Autodesk Inventor part; units mm, degrees
ref_plane "YZ Plane" through (0, 0, 0) normal (1, 0, 0) x (0, 1, 0)
ref_plane "XZ Plane" through (0, 0, 0) normal (0, 1, 0) x (-1, 0, 0)
ref_plane "XY Plane" through (0, 0, 0) normal (0, 0, 1) x (1, 0, 0)
sketch "Sketch1" plane through (0, 0, 0) normal (0, 0, 1) x (1, 0, 0)
  arc A0 (-5, -2.9) -> (-4.8506, -3.2565) centre (-4.5, -2.9) ccw
  line L0 (-5, -2.6) -> (-5, -2.9)
  arc A1 (-4.5, -2.1) -> (-5, -2.6) centre (-4.5, -2.6) ccw
  line L1 (-4.8506, -3.2565) -> (-1.8506, -6.2065)
  arc A2 (-1.8506, -6.2065) -> (-1.5, -6.35) centre (-1.5, -5.85) ccw
  line L2 (-1.5, -6.35) -> (1.5, -6.35)
  line L3 (4.5, -2.1) -> (-4.5, -2.1)
  arc A3 (1.5, -6.35) -> (1.8506, -6.2065) centre (1.5, -5.85) ccw
  line L4 (4.8506, -3.2565) -> (1.8506, -6.2065)
  arc A4 (5, -2.6) -> (4.5, -2.1) centre (4.5, -2.6) ccw
  arc A5 (4.8506, -3.2565) -> (5, -2.9) centre (4.5, -2.9) ccw
  line L5 (5, -2.6) -> (5, -2.9)
  line L6 (-2.5, 0) -> (2.5, 0)
  line L7 (-2.5, 0) -> (-2.5, -2.1)
  line L8 (2.5, 0) -> (2.5, -2.1)
  point P0 (0, -6.35)
  point P1 (0, 0)
  point P2 (0, -2.1)
  point P3 (0, 0)
  dimension "d9" = 4.25
  dimension "d10" = 10
  dimension "d12" = 0.3
  dimension "d13" = 9
  dimension "d14" = 3
  dimension "d17" = 2.1
  dimension "d18" = 5
extrude "Extrusion1" add sketch "Sketch1" along normal blind 8
sketch "Sketch2" plane through (0, 0, 0) normal (0, 0, -1) x (-1, 0, 0)
  line L0 (-2.5, 0) -> (2.5, 0)
  line L1 (2.5, 0) -> (12, 0)
  line L2 (-2.5, -2.1) -> (-2.5, 0)
  line L3 (12, 0) -> (3.3532, 8.6468)
  line L4 (-0.6066, 4.687) -> (2.0804, 2)
  line L5 (3.3532, 8.6468) -> (-0.6066, 4.687)
  line L6 (2.0804, 2) -> (6.0402, 5.9598)
  line L7 (10, 0) -> (10, 2)
  line L8 (3.3532, 8.6468) -> (1.2319, 10.7681)
  line L9 (1.2319, 10.7681) -> (-4.8492, 4.687)
  line L10 (-4.8492, 4.687) -> (-2.5, 0)
  point P0 (0, 0)
  dimension "d21" = 12
  dimension "d23" = 45
  dimension "d24" = 3.8
  dimension "d25" = 5.6
  dimension "d26" = 2
  dimension "d28" = 3
  dimension "d34" = 10
extrude "Extrusion2" add sketch "Sketch2" against normal up to surface (8 mm away) contours L10 L9 L8 L5 L4 L6 L3 L7 L1 L0 | L3 L6 L4 L5
sketch "Sketch3" plane through (-1.2319, 10.7681, 0) normal (-0.7071, 0.7071, 0) x (-0.7071, -0.7071, 0)
  line L0 (12.4, 0) -> (12.4, 8)
  line L1 (6.8, 0) -> (3, 0)
  line L2 (12.4, 0) -> (0, 0)
  circle A0 centre (4.9, 4) radius 1.9
  point P0 (6.7431, 0)
  point P1 (12.4, 4)
  point P2 (4.9, 0)
  dimension "d31" = 3.8
extrude "Extrusion3" cut sketch "Sketch3" against normal blind 5.6
properties part number "Profil-ElBoardHold"
The listing builds one solid part. Answer for the finished solid, in the listing's coordinates (mm). A direction names the side the tool comes from. Give positions to 0.01 mm unless a question says otherwise; leave off trailing zeros. Write each loop counter-clockwise with the first axis right and the second up, starting at its lowest first coordinate (ties: lowest second). Pieces come first, ordered by that corner, then holes. Notation, with made-up numbers: (-16.75, 4) - (6.25, 4) arc R17 cw to (6.25, 33) - close; hole circle Ø1 at (39, 30.25). An arc over 180 degrees is marked (long way). Use a Markdown table: item, result.
1. Section A-A on z = 7.5 is taken. Write down the section's boundary in (x, y).
Values follow:
| item | result |
|---|---|
| outline | (-10, 0) - (-2.5, 0) - (-2.5, -2.1) - (-4.5, -2.1) arc R0.5 ccw to (-5, -2.6) - (-5, -2.9) arc R0.5 ccw to (-4.85, -3.26) - (-1.85, -6.21) arc R0.5 ccw to (-1.5, -6.35) - (1.5, -6.35) arc R0.5 ccw to (1.85, -6.21) - (4.85, -3.26) arc R0.5 ccw to (5, -2.9) - (5, -2.6) arc R0.5 ccw to (4.5, -2.1) - (2.5, -2.1) - (2.5, 0) - (4.85, 4.69) - (-1.23, 10.77) - (-10, 2) - close |
2. Each of these flat-tipped pins is pushed along its axis until it touches: P1, Ø0.6, axis at y = -1, z = 2, coming from the -X side; P2, Ø0.6, axis at x = 3, z = 2.5, coming from the +Y side; P3, Ø2, axis at x = 3.5, z = 1.5, coming from the +Y side. Where does it stop, or does it pass through?
Values follow:
| item | result |
|---|---|
| P1 | stops at x = -2.5 |
| P2 | stops at y = 6.84 |
| P3 | stops at y = 7.04 |
3. Section B-B on y = 1 is taken. Write down the section's boundary in (x, z).
Values follow:
| item | result |
|---|---|
| outline | (-10, 0) - (3, 0) - (3, 8) - (-10, 8) - close |
4. Find the intervals of material crossed by probe 1 along X at (y, z) = (-1.5, 3.75); probe 2 along Y at (x, z) = (-7, 2.25); probe 3 along Y at (x, z) = (-3.75, 7.25), in increasing order. Write a range as from..to.
Values follow:
| item | result |
|---|---|
| probe 1 | x = -2.5..2.5 |
| probe 2 | y = 0..5 |
| probe 3 | y = -4.34..-2.1, 0..8.25 |
5. A tool of negligible diameter and unlimited length cuts with its end or side. For faces 4 (the flat face through (3.691, 2.376, 3.944)), 5 (the flat face through (-6, 0, 4)), 6 (the flat face through (-0.72, 3.36, 4.03)), from which of +Z, -Z, +X, -X, +Y, -Y can it reach the whole face along a straight path? Write none if from no direction.
Values follow:
| item | result |
|---|---|
| face 4 | +Z, -Z, +X |
| face 5 | +Z, -Z, -X |
| face 6 | none |
6. Section D-D on x = 2.25 is taken. Write down the section's boundary in (y, z), plus the area to 3 significant figures.
Values follow:
| item | result |
|---|---|
| outline | (-5.81, 0) - (7.29, 0) - (7.29, 8) - (-5.81, 8) - close |
| area | 105 mm² |
7. Section C-C on z = 3.75 is taken. Write down the section's boundary in (x, y), plus the area to 3 significant figures.
Values follow:
| item | result |
|---|---|
| outline | (-10, 0) - (-2.5, 0) - (-2.5, -2.1) - (-4.5, -2.1) arc R0.5 ccw to (-5, -2.6) - (-5, -2.9) arc R0.5 ccw to (-4.85, -3.26) - (-1.85, -6.21) arc R0.5 ccw to (-1.5, -6.35) - (1.5, -6.35) arc R0.5 ccw to (1.85, -6.21) - (4.85, -3.26) arc R0.5 ccw to (5, -2.9) - (5, -2.6) arc R0.5 ccw to (4.5, -2.1) - (2.5, -2.1) - (2.5, 0) - (4.85, 4.69) - (-1.23, 10.77) - (-3.36, 8.64) - (0.6, 4.67) - (-2.07, 2.01) - (-6.03, 5.97) - (-10, 2) - close |
| area | 119 mm² |
8. For a pull along X with two mould halves and no side action, classify faces 1 (the flat face through (-3.37, -4.71, 3.94)), 2 (the flat face through (2.5, -1, 4)), 3 (the cylindrical face through (-3.47, 4.63, 5.6)) as released by +X, released by -X, zero draft, split by the parting line, or undercut.
Values follow:
| item | result |
|---|---|
| face 1 | released by -X |
| face 2 | released by +X |
| face 3 | undercut |
